Read the model definition and answer for the solid it produces. Units are mm, in the model's axes. Face numbers are marked on the shaded views. A direction names the side the tool comes from. Give positions to 0.01 mm unless a question says otherwise; leave off trailing zeros. Order: outer loops, then holes, each group sorted by start corner. A loop starts at its lowest first (then second) coordinate and runs counter-clockwise, first axis right, second up.
Item 1: A cutting plane is placed at D-D (y = 46). Write down the section's boundary in (x, z).
Item 2: Given pin 1 Ø8 at (x, z) = (-45, -20) entering from +Y; pin 2 Ø12.5 at (y, z) = (19, -33.5) entering from +X; pin 3 Ø3 at (y, z) = (47.5, -13) entering from -X; pin 4 Ø17 at (x, y) = (-58.76, 25.4) entering from -Z, each flat-ended and moving along its own axis, determine where each tip first touches the part or whether it passes through.
Item 3: A cutting plane is placed at C-C (z = -29.5). Write down the section's boundary in (x, y).
Item 4: Find the intervals of material crossed by line 1 along Z through (x, y) = (-33.5, 36); line 2 along X through (y, z) = (19.5, -20); line 3 along Y through (x, z) = (-49, -28), in increasing order.
Item 5: A cutting plane is placed at B-B (x = -84). Write down the section's boundary in (y, z), plus the area to 3 significant figures.
Item 6: A cutting plane is placed at A-A (y = 25.4). Write down the section's boundary in (x, z), plus the area to 3 significant figures.
Item 7: The mould has two halves that part along Z. Classify the marked faces 4, 5 and 6: +Z half, -Z half, draft (parallel to the pull), parting line (faces both ways), or undercut.
Item 8: Which of the six approach directions +Z, -Z, +X, -X, +Y, -Y give full straight-line access (tool end or side, diameter ignored) to the marked faces 1, 2 and 3?
from build123d import *

# Parameters (mm, degrees)
SKETCH1_W           = 91.948
SKETCH1_H           = 38.1
BOSS_EXTRUDE1_DEPTH = 50.8
SKETCH2_R           = 9.525
CUT_EXTRUDE1_DEPTH  = 116.82034416
SKETCH3_W           = 19.05
SKETCH3_H           = 12.7
CUT_EXTRUDE2_DEPTH  = 116.82034416
SKETCH4_W           = 12.7
SKETCH4_H           = 25.4
SKETCH4_W_2         = 72.898
CUT_EXTRUDE5_DEPTH  = 44.45
CUT_EXTRUDE6_DEPTH  = 116.82034416


with BuildPart() as part:
    # Sketch1 → Boss-Extrude1 (new body)
    with BuildSketch(Plane(origin=(0, 0, 0), x_dir=(1, 0, 0), z_dir=(0, 1, 0))):
        with Locations((-50.887251908, 28.561750636)):
            Rectangle(SKETCH1_W, SKETCH1_H)
    extrude(amount=BOSS_EXTRUDE1_DEPTH)

    # Sketch2 → Cut-Extrude1 (cut, through all)
    with BuildSketch(Plane.XY.offset(-9.511750636)):
        with Locations((-58.761251908, 25.4)):
            Circle(SKETCH2_R)
    extrude(amount=-CUT_EXTRUDE1_DEPTH, mode=Mode.SUBTRACT)

    # Sketch3 → Cut-Extrude2 (cut, through all)
    with BuildSketch(Plane.XY.offset(-9.511750636)):
        with Locations((-87.336251908, 44.45)):
            Rectangle(SKETCH3_W, SKETCH3_H)
    extrude(amount=-CUT_EXTRUDE2_DEPTH, mode=Mode.SUBTRACT)

    # Sketch4 → Cut-Extrude5 (cut)
    with BuildSketch(Plane(origin=(0, 50.8, 0), x_dir=(1, 0, 0), z_dir=(0, 1, 0))):
        with Locations((-84.161251908, 28.561750636)):
            Rectangle(SKETCH4_W, SKETCH4_H)
        with Locations((-41.362251908, 28.561750636)):
            Rectangle(SKETCH4_W_2, SKETCH4_H)
    extrude(amount=-CUT_EXTRUDE5_DEPTH, mode=Mode.SUBTRACT)

    # Sketch5 → Cut-Extrude6 (cut, through all)
    with BuildSketch(Plane.XY.offset(-9.511750636)):
        Polygon((-23.888342421, 32.865820845), (-4.913251908, 0), (-4.913251908, 50.8), (-54.951251908, 50.8), align=None)
    extrude(amount=-CUT_EXTRUDE6_DEPTH, mode=Mode.SUBTRACT)


solid = part.part
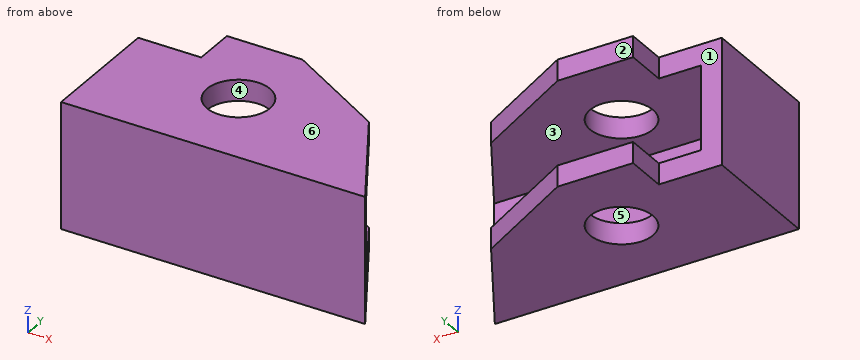
Response values:
1. outline: (-77.81, -47.61) - (-46.64, -47.61) - (-46.64, -41.26) - (-77.81, -41.26) - close; (-77.81, -15.86) - (-46.64, -15.86) - (-46.64, -9.51) - (-77.81, -9.51) - close
2. pin 1: stops at y = 6.35
2. pin 2: stops at x = -90.51
2. pin 3: stops at x = -77.81
2. pin 4: passes through
3. outline: (-96.86, 0) - (-4.91, 0) - (-8.58, 6.35) - (-90.51, 6.35) - (-90.51, 38.1) - (-96.86, 38.1) - close
4. line 1: z = -47.61 to -41.26, -15.86 to -9.51
4. line 2: x = -96.86 to -90.51
4. line 3: y = 0 to 6.35
5. outline: (0, -47.61) - (38.1, -47.61) - (38.1, -41.26) - (6.35, -41.26) - (6.35, -15.86) - (38.1, -15.86) - (38.1, -9.51) - (0, -9.51) - close
5. area: 645 mm2
6. outline: (-96.86, -47.61) - (-68.29, -47.61) - (-68.29, -41.26) - (-90.51, -41.26) - (-90.51, -15.86) - (-68.29, -15.86) - (-68.29, -9.51) - (-96.86, -9.51) - close; (-49.24, -47.61) - (-19.58, -47.61) - (-19.58, -41.26) - (-49.24, -41.26) - close; (-49.24, -15.86) - (-19.58, -15.86) - (-19.58, -9.51) - (-49.24, -9.51) - close
6. area: 901 mm2
7. face 4: draft
7. face 5: undercut
7. face 6: +Z half
8. face 1: +Z, -Z, -X, +Y
8. face 2: +Z, -Z, +X, -X, +Y
8. face 3: +X, +Y
